Autodesk Inventor part; units mm, degrees
ref_plane "YZ Plane" through (0, 0, 0) normal (1, 0, 0) x (0, 1, 0)
ref_plane "XZ Plane" through (0, 0, 0) normal (0, 1, 0) x (-1, 0, 0)
ref_plane "XY Plane" through (0, 0, 0) normal (0, 0, 1) x (1, 0, 0)
sketch "Esquisse3" plane through (0, 0, 0) normal (0, 0, 1) x (1, 0, 0)
  line L0 (0, 0) -> (25.2376, 0)
  line L1 (25.2376, 0) -> (25.2376, 58.756)
  line L2 (25.2376, 58.756) -> (25.2376, 118.9226)
  line L3 (25.2376, 118.9226) -> (11.8572, 160.0383)
  line L4 (11.8572, 160.0383) -> (11.8572, 201.5839)
  line L5 (0, 244.1266) -> (0, -47.634)
  line L6 (13.8572, 201.5839) -> (13.8572, 160.3556)
  line L7 (13.8572, 160.3556) -> (27.2376, 119.2398)
  line L8 (27.2376, 119.2398) -> (27.2376, 58.756)
  line L9 (27.2376, 58.756) -> (27.2376, -2)
  line L10 (27.2376, -2) -> (0, -2)
  line L11 (11.8572, 201.5839) -> (13.8572, 201.5839)
  line L12 (25.2376, 0) -> (27.2376, 0)
  dimension "d2" = 58.756
  dimension "d3" = 90
  dimension "d4" = 2
revolve "Révolution1" add sketch "Esquisse3" angle 360 about axis through (0, 244.1266, 0) along (0, -1, 0) contours L1 L2 L3 L4 L11 L6 L7 L8 L9 L12
sketch "Esquisse4" plane through (0, 0, 0) normal (0, -1, 0) x (1, 0, 0)
  circle A0 centre (0, 0) radius 25.2376
  circle A1 centre (0, 0) radius 27.1886
extrude "Extrusion1" add sketch "Esquisse4" along normal blind 23.5
Design review of the part built by this model. Coordinates are the model's own, in mm. Round coordinates to 2 decimals unless told otherwise and drop trailing zeros. Order: outer loops, then holes, each group sorted by start corner. A loop starts at its lowest first (then second) coordinate and runs counter-clockwise, first axis right, second up. Notation, with made-up numbers: (34, 87) - (64, 87) arc R22 cw to (64, 111) - close; hole circle Ø8 at (69, -36.5). An arc over 180 degrees is marked (long way). Return JSON: item names as keys, results as strings.
Q1. Consider section A-A on x = 0. Write out the cut boundary in (y, z).
Computed values:
{"outline": "(-23.5, -27.19) - (0, -27.19) - (0, -27.24) - (119.24, -27.24) - (160.36, -13.86) - (201.58, -13.86) - (201.58, -11.86) - (160.04, -11.86) - (118.92, -25.24) - (-23.5, -25.24) - close; (-23.5, 25.24) - (118.92, 25.24) - (160.04, 11.86) - (201.58, 11.86) - (201.58, 13.86) - (160.36, 13.86) - (119.24, 27.24) - (0, 27.24) - (0, 27.19) - (-23.5, 27.19) - close"}
Q2. The part is to be moulded in two halves that separate along X. For faces 1 (the flat face through (-6.2, 201.584, 10.3)), 2 (the conical face through (-13.61, 143.76, -10.44)), 3 (the cylindrical face through (-20.028, 48.708, 15.357)), 4 (the cylindrical face through (25.16, 58.79, -10.43)), say which applies: pulls with the +X half, pulls with the -X half, needs draft (parallel to the pull), parting line crosses it, or undercut.
Computed values:
{"face 1": "needs draft", "face 2": "undercut", "face 3": "undercut", "face 4": "parting line crosses it"}
Q3. For pin 1 Ø5 at (x, y) = (2.5, 135.5) entering from -Z; pin 2 Ø5 at (x, y) = (-13, 22) entering from +Z; pin 3 Ø5 at (x, z) = (13, 8.5) entering from +Y; pin 4 Ø5 at (x, y) = (-7, 40.5) entering from -Z, all flat-tipped, find the tip position at first contact; note any pin that passes through.
Computed values:
{"pin 1": "stops at z = -22.66", "pin 2": "stops at z = 25.13", "pin 3": "stops at y = 201.58", "pin 4": "stops at z = -26.86"}
Q4. Consider section C-C on y = 59. Write out the cut boundary in (x, z).
Computed values:
{"outline": "circle Ø54.48 at (0, 0); hole circle Ø50.48 at (0, 0)"}
Q5. Consider section B-B on z = 0. Write out the cut boundary in (x, y).
Computed values:
{"outline": "(-27.24, 0) - (-27.19, 0) - (-27.19, -23.5) - (-25.24, -23.5) - (-25.24, 118.92) - (-11.86, 160.04) - (-11.86, 201.58) - (-13.86, 201.58) - (-13.86, 160.36) - (-27.24, 119.24) - close; (11.86, 160.04) - (25.24, 118.92) - (25.24, -23.5) - (27.19, -23.5) - (27.19, 0) - (27.24, 0) - (27.24, 119.24) - (13.86, 160.36) - (13.86, 201.58) - (11.86, 201.58) - close"}
Q6. Wall thickness on L1, parallel to Z at x = 0, y = 87; L2, parallel to Z at x = 0, y = 172; L3, parallel to X at y = 49, z = 10: over which ranges is each line inside the solid? List them lowest first. Write a range as [from, to].
Computed values:
{"L1": "z = [-27.24, -25.24], [25.24, 27.24]", "L2": "z = [-13.86, -11.86], [11.86, 13.86]", "L3": "x = [-25.34, -23.17], [23.17, 25.34]"}
